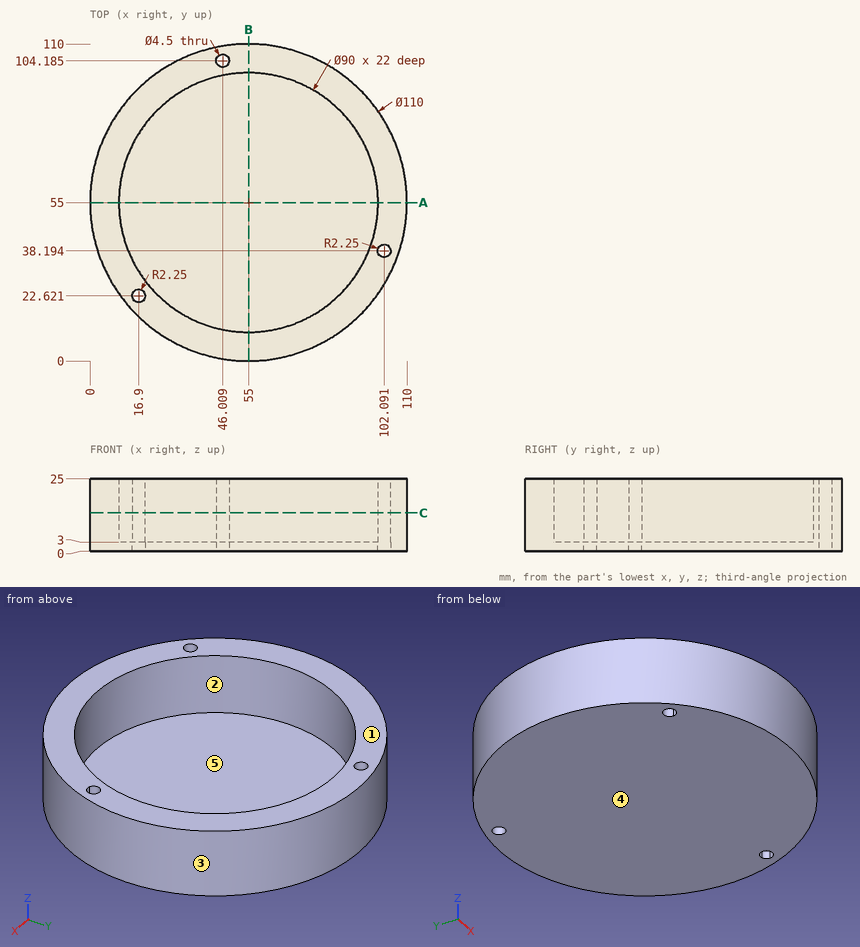
The drawing under review shows one solid part. Ordinate dimensions are in mm from its lowest x, y, z. A direction names the side the tool comes from. Round coordinates to 2 decimals unless told otherwise and drop trailing zeros. Write each loop counter-clockwise with the first axis right and the second up, starting at its lowest first coordinate (ties: lowest second). Pieces come first, ordered by that corner, then holes.
(1) Mouldability with a two-part tool opening along X and no side actions: class the marked faces 1, 2 and 3 as +X half, -X half, draft (parallel to the pull), parting line (faces both ways), or undercut.
(2) We need section C-C on z = 13.25. Give the number of separate pieces and of enclosed holes in the cut face, and give its area (3 significant figures).
(3) We need section A-A on y = 55. Give the boundary of the cut face in (x, z), and give its area (3 significant figures).
(4) Wall thickness on L1, parallel to Y at x = 55.5, z = 16.5; L2, parallel to X at y = 23, z = 9 (1 decimal): over which ranges is each line inside the solid? List them lowest first.
(5) Machinability: for the marked faces 4 and 5, which of the approach directions +Z, -Z, +X, -X, +Y, -Y give a long, thin tool a straight path to every point of the face, cutting with its end or side? Answer none if there is none.
(6) Insertion check: pin 1 (1.5 mm diameter, centred on x = 66.5, z = 17, fed in from -Y); pin 2 (10 mm diameter, centred on x = 20.5, z = 22, fed in from +Y); pin 3 (12 mm diameter, centred on x = 75.5, z = 21.5, fed in from +Y) (1 decimal); pin 4 (2.5 mm diameter, centred on x = 46.01, y = 104.19, fed in from -Z). Each pin has a flat end and moves straight along its axis. Give the tip position at first contact, or say it passes through.
Findings below:
1. face 1: draft
1. face 2: undercut
1. face 3: parting line
2. separate pieces: 1
2. enclosed holes: 4
2. area: 3,090 mm2
3. outline: (0, 0) - (110, 0) - (110, 25) - (100, 25) - (100, 3) - (10, 3) - (10, 25) - (0, 25) - close
3. area: 770 mm2
4. L1: y = 0 to 10, 100 to 110
4. L2: x = 10.3 to 14.7, 19.1 to 23.4, 86.6 to 99.7
5. face 4: -Z, +X, -X, +Y, -Y
5. face 5: +Z
6. pin 1: stops at y = 1.06
6. pin 2: stops at y = 101.42
6. pin 3: stops at y = 108.1
6. pin 4: passes through
